from build123d import *

# Parameters (mm, degrees)
BOSS_EXTRUDE1_DEPTH      = 1.5
BOSS_EXTRUDE2_DEPTH      = 1
SKETCH4_R                = 4.75
CUT_EXTRUDE1_DEPTH       = 23.898325822
SKETCH5_W                = 17.56
SKETCH5_H                = 2.5
BOSS_EXTRUDE3_DEPTH      = 0.15
SKETCH6_W                = 17.56
SKETCH6_H                = 2.5
BOSS_EXTRUDE4_DEPTH      = 11.35
SKETCH7_W                = 2.5
SKETCH7_H                = 2.4
BOSS_EXTRUDE5_DEPTH      = 12.72
BOSS_EXTRUDE6_DEPTH      = 0.8
BOSS_EXTRUDE6_DEPTH_BACK = 1.3
SKETCH9_W                = 1.40416608
SKETCH9_H                = 2.4
BOSS_EXTRUDE7_DEPTH      = 0.8
CHAMFER3_SIZE            = 1.039230485
CHAMFER3_SIZE_2          = 1.8
BOSS_EXTRUDE8_DEPTH      = 1.2


with BuildPart() as part:
    # Sketch1 → Boss-Extrude1 (new body)
    with BuildSketch(Plane.XY):
        with BuildLine():
            ThreePointArc((14.980604809, 6.55), (8.78, 2), (2.579395191, 6.55))
            Line((2.579395191, 6.55), (0, 6.55))
            Line((0, 6.55), (0, 0))
            Line((0, 0), (17.56, 0))
            Line((17.56, 0), (17.56, 6.55))
            Line((17.56, 6.55), (14.980604809, 6.55))
        make_face()
        with BuildLine():
            ThreePointArc((2.579395191, 6.55), (2.679421093, 10.743420825), (5.32, 14.002581212))
            Line((5.32, 14.002581212), (5.32, 14.619498126))
            ThreePointArc((5.32, 14.619498126), (1.449679407, 11.382680416), (0, 6.55))
            Line((0, 6.55), (2.579395191, 6.55))
        make_face()
        with BuildLine():
            ThreePointArc((12.24, 14.002581212), (14.880578907, 10.743420825), (14.980604809, 6.55))
            Line((14.980604809, 6.55), (17.56, 6.55))
            ThreePointArc((17.56, 6.55), (16.110320593, 11.382680416), (12.24, 14.619498126))
            Line((12.24, 14.619498126), (12.24, 14.002581212))
        make_face()
    extrude(amount=BOSS_EXTRUDE1_DEPTH)

    # Sketch3 → Boss-Extrude2 (add)
    with BuildSketch(Plane.XY.offset(1.5)):
        with BuildLine():
            Line((12.24, 14.619498126), (12.24, 14.002581212))
            ThreePointArc((12.24, 14.002581212), (8.78, 2), (5.32, 14.002581212))
            Line((5.32, 14.002581212), (5.32, 14.619498126))
            ThreePointArc((5.32, 14.619498126), (1.449679407, 11.382680416), (0, 6.55))
            Line((0, 6.55), (0, 0))
            Line((0, 0), (17.56, 0))
            Line((17.56, 0), (17.56, 6.55))
            ThreePointArc((17.56, 6.55), (16.110320593, 11.382680416), (12.24, 14.619498126))
        make_face()
        with BuildLine():
            Line((5.32, 14.619498126), (12.24, 14.619498126))
            Line((12.24, 14.619498126), (12.24, 14.002581212))
            ThreePointArc((12.24, 14.002581212), (8.78, 2), (5.32, 14.002581212))
            Line((5.32, 14.002581212), (5.32, 14.619498126))
        make_face()
    extrude(amount=BOSS_EXTRUDE2_DEPTH)

    # Sketch4 → Cut-Extrude1 (cut, through all)
    with BuildSketch(Plane(origin=(0, 0, 1.5), x_dir=(-1, 0, 0), z_dir=(0, 0, -1))):
        with Locations((-8.78, 8.5)):
            Circle(SKETCH4_R)
    extrude(amount=-CUT_EXTRUDE1_DEPTH, mode=Mode.SUBTRACT)

    # Sketch5 → Boss-Extrude3 (add)
    with BuildSketch(Plane.XZ):
        with Locations((8.78, 1.25)):
            Rectangle(SKETCH5_W, SKETCH5_H)
    extrude(amount=BOSS_EXTRUDE3_DEPTH)

    # Sketch6 → Boss-Extrude4 (add)
    with BuildSketch(Plane.XZ.offset(0.15)):
        with Locations((8.78, 1.25)):
            Rectangle(SKETCH6_W, SKETCH6_H)
    extrude(amount=BOSS_EXTRUDE4_DEPTH)

    # Sketch7 → Boss-Extrude5 (add)
    with BuildSketch(Plane.ZY):
        with Locations((1.25, -10.3)):
            Rectangle(SKETCH7_W, SKETCH7_H)
    extrude(amount=BOSS_EXTRUDE5_DEPTH)

    # Sketch8 → Boss-Extrude6 (add, two sides: drawn at the far end of the back side and taken through both)
    with BuildSketch(Plane(origin=(0, 0, 0), x_dir=(-1, 0, 0), z_dir=(0, 0, -1)).offset(-BOSS_EXTRUDE6_DEPTH_BACK)):
        Polygon((13.121190309, -9.1), (13.375962235, -5.8), (14.472698599, -5.884672011), (11.85625922, -2.1), (11.31583392, -9.1), (12.72, -9.1), (12.72, -11.5), align=None)
    extrude(amount=BOSS_EXTRUDE6_DEPTH + BOSS_EXTRUDE6_DEPTH_BACK)

    # Sketch9 → Boss-Extrude7 (add)
    with BuildSketch(Plane(origin=(0, 0, 0), x_dir=(-1, 0, 0), z_dir=(0, 0, -1))):
        with Locations((12.01791696, -10.3)):
            Rectangle(SKETCH9_W, SKETCH9_H)
    extrude(amount=BOSS_EXTRUDE7_DEPTH)

    # Chamfer3
    # the kernel refuses this chamfer: 1.8, 1.039230485 mm, written as the material it adds along each edge
    with BuildSketch(Plane(origin=(-11.31583392, -11.5, 0), x_dir=(-0.05789386240267112, 0, -0.9983227437537925), z_dir=(0, 1, 0))) as chamfer3_piece_1_section:
        Polygon((CHAMFER3_SIZE * 0.998322743313, -CHAMFER3_SIZE * 0.0578938623771), (-CHAMFER3_SIZE_2 * 0.0578938624027, -CHAMFER3_SIZE_2 * 0.998322743754), (0, 0), align=None)
    chamfer3_piece_1 = extrude(amount=2.4, mode=Mode.PRIVATE)
    chamfer3_piece_1 = split(chamfer3_piece_1, bisect_by=Plane(origin=(-11.20125383, -10.584128582, -0.396089169), z_dir=(-0.9970330575262718, -0.07697455553502185, 0)), keep=Keep.TOP, mode=Mode.PRIVATE)
    chamfer3_piece_1 = split(chamfer3_piece_1, bisect_by=Plane(origin=(-11.276211274, -10.589915567, -0.8), z_dir=(0, 0, 1)), keep=Keep.TOP, mode=Mode.PRIVATE)
    add(chamfer3_piece_1)
    with BuildSketch(Plane(origin=(-11.31583392, -11.5, 0), x_dir=(-0.05789386240267112, 0, -0.9983227437537925), z_dir=(0, 1, 0))) as chamfer3_piece_2_section:
        Polygon((CHAMFER3_SIZE * 0.998322743313, -CHAMFER3_SIZE * 0.0578938623771), (-CHAMFER3_SIZE_2 * 0.0578938624027, -CHAMFER3_SIZE_2 * 0.998322743754), (0, 0), align=None)
    chamfer3_piece_2 = extrude(amount=2.4, mode=Mode.PRIVATE)
    chamfer3_piece_2 = split(chamfer3_piece_2, bisect_by=Plane(origin=(-11.222198101, -10.312842427, -0.281258227), z_dir=(0.9970330575262718, 0.07697455553502185, 0)), keep=Keep.TOP, mode=Mode.PRIVATE)
    chamfer3_piece_2 = split(chamfer3_piece_2, bisect_by=Plane(origin=(-10.603533265, -10.265079266, -0.8), z_dir=(0, 0, 1)), keep=Keep.TOP, mode=Mode.PRIVATE)
    add(chamfer3_piece_2)

    # Sketch10 → Boss-Extrude8 (add)
    with BuildSketch(Plane.XY.offset(1.3)):
        Polygon((-12.72, -11.5), (-12.72, -9.1), (-13.121190309, -9.1), align=None)
    extrude(amount=BOSS_EXTRUDE8_DEPTH)


solid = part.part
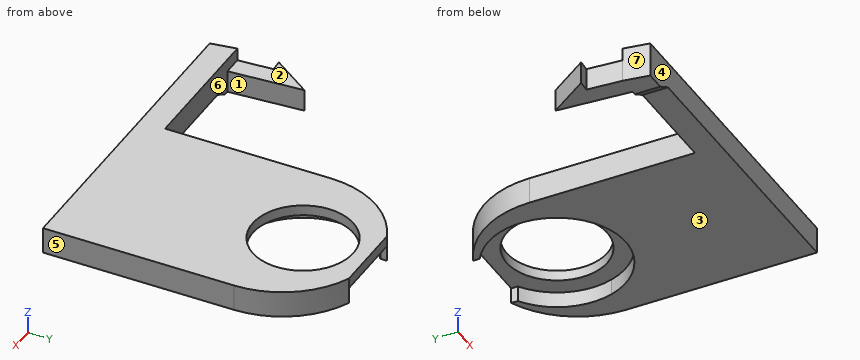
Could you check a few things on this model? Use its own coordinates, in mm. Face numbers are marked on the shaded views. A direction names the side the tool comes from. Coordinates: 2 decimals unless noted, no trailing zeros. Order: outer loops, then holes, each group sorted by start corner. A loop starts at its lowest first (then second) coordinate and runs counter-clockwise, first axis right, second up. Notation, with made-up numbers: (22.25, -7.75) - (27.25, -7.75) arc R20 ccw to (27.25, 1.25) - close; hole circle Ø3 at (7.5, 5.5). An arc over 180 degrees is marked (long way). Answer in a Markdown table with one row per item. Add a question column.
(1) On a 3-axis mill with a long thin cutter (end or side, diameter ignored), from which of +Z, -Z, +X, -X, +Y, -Y can I reach the whole of each face in a straight line? I mean the marked faces 1, 2 and 3. Say none if no direction works.
(2) If we section it at D-D, the plane x = -7: Please give me the cut outline in (y, z), then the cut area to 3 significant figures.
(3) Will these pins go through, and if not, where does the flat tip stop? pin 1 (1.6 mm diameter, centred on x = -9.5, z = 1, fed in from +Y); pin 2 (5 mm diameter, centred on x = 1.5, y = -7, fed in from -Z); pin 3 (2.5 mm diameter, centred on x = -13, y = -7, fed in from +Z).
(4) If we section it at B-B, the plane z = 1.95: Please give me the cut outline in (x, y), then the cut area to 3 significant figures.
(5) If we section it at C-C, the plane y = -4.5: Please give me the cut outline in (x, z).
(6) If we section it at A-A, the plane x = 8.78: Please give me the cut outline in (y, z), then the cut area to 3 significant figures.
(7) I need wall thicknesses on L1, parallel to Y at x = 8.78, z = 1.8; L2, parallel to Y at x = -7.5, z = 1.6; L3, parallel to X at y = 11, z = 2.3. Which ranges of each line are inside material? Lowest first, please.
(8) If we mould it in two halves opening along X, with no side actions, what happens to the marked faces 4, 5, 6 and 7? For each: released by +X, released by -X, zero draft, split by the parting line, or undercut.
Results are:
| question | item | result |
|---|---|---|
| 1 | face 1 | +Z, -Z, +Y |
| 1 | face 2 | +Z, -X, +Y |
| 1 | face 3 | -Z, +X, +Y, -Y |
| 2 | outline | (-11.5, 0) - (-9.1, 0) - (-9.1, 2.5) - (-11.5, 2.5) - close |
| 2 | area | 6.00 mm2 |
| 3 | pin 1 | stops at y = -9.1 |
| 3 | pin 2 | stops at z = 0 |
| 3 | pin 3 | stops at z = 1.3 |
| 4 | outline | (-13.12, -9.1) - (-12.72, -11.5) - (17.56, -11.5) - (17.56, 6.55) arc R8.78 ccw to (12.24, 14.62) - (5.32, 14.62) arc R8.78 ccw to (0, 6.55) - (0, -9.1) - close; hole circle Ø9.5 at (8.78, 8.5) |
| 4 | area | 395 mm2 |
| 5 | outline | (-13.52, -0.8) - (-11.67, -0.8) - (-11.67, 1.3) - (-13.52, 1.3) - close; (0, 0) - (17.56, 0) - (17.56, 2.5) - (0, 2.5) - close |
| 6 | outline | (-11.5, 0) - (2, 0) - (2, 1.5) - (3.75, 1.5) - (3.75, 2.5) - (-11.5, 2.5) - close; (13.25, 1.5) - (14.62, 1.5) - (14.62, 2.5) - (13.25, 2.5) - close |
| 6 | area | 36.9 mm2 |
| 7 | L1 | y = -11.5 to 3.75, 13.25 to 14.62 |
| 7 | L2 | y = -11.5 to -9.1 |
| 7 | L3 | x = 1.21 to 4.74, 12.82 to 16.35 |
| 8 | face 4 | zero draft |
| 8 | face 5 | released by +X |
| 8 | face 6 | undercut |
| 8 | face 7 | released by -X |
